The model under review builds one solid part; all positions refer to its coordinate system, in mm. A direction names the side the tool comes from. Round coordinates to 2 decimals unless told otherwise and drop trailing zeros. Write each loop counter-clockwise with the first axis right and the second up, starting at its lowest first coordinate (ties: lowest second). Pieces come first, ordered by that corner, then holes. Notation, with made-up numbers: M 13.25,61.25 L 36.25,61.25 A24 cw 36.25,100.25 Z; hole C 30.5,17.5 d9. An arc over 180 degrees is marked long. One line per item, written item: value. Start each with the question number.
1) Wall thickness on probe 1 along Z at (x, y) = (0, -85); probe 2 along Y at (x, z) = (16, 29); probe 3 along X at (y, z) = (-97, -0.5): over which ranges is each line inside the solid? List them lowest first.
2) Mouldability with a two-part tool opening along Z and no side actions: class faces 3 (the face through (0, -30, 0)), 4 (the face through (-2.927, -69.44, -13.183)), 5 (the face through (51.884, -15.21, -53.401)), 6 (the face through (0, 0, -2)) as +Z half, -Z half, draft (parallel to the pull), parting line (faces both ways), or undercut.
3) For P1, Ø3, axis at x = 11, y = -62, coming from the -Z side; P2, Ø1.5, axis at y = -51.5, z = 2.5, coming from the -X side; P3, Ø4, axis at x = 6, y = -80, coming from the -Z side, all flat-tipped, find the tip position at first contact; note any pin that passes through.
4) Tool access review of faces 1 (the face through (51.962, -15.21, 48.431)), 2 (the face through (-6.68, -39.86, -30.08)): name each direction out of +Z, -Z, +X, -X, +Y, -Y from which nothing blocks a thin tool from reaching the whole face with its end or side.
5) Take a section at D-D, the plane z = -22. Write out the cut boundary in (x, y), and give its area (3 significant figures).
6) Take a section at B-B, the plane x = 0. Write out the cut boundary in (y, z), and give its area (3 significant figures).
7) Take a section at A-A, the plane z = 0. Write out the cut boundary in (x, y), and give its area (3 significant figures).
8) Take a section at C-C, the plane y = -99.5. Write out the cut boundary in (x, z).
from build123d import *

# Parameters (mm, degrees)
F0_W     = 105.912518
F0_H     = 104.761295
F1_DEPTH = 30
F2_R     = 5
F3_R     = 30.813713
F3_R_2   = 23.380782
F4_DEPTH = 20
F5_R     = 23.490351
F5_R_2   = 13.503853
F6_DEPTH = 80


with BuildPart() as f1:
    # F0 (on Front) → F1 (new body)
    with BuildSketch(Plane.XZ):
        with Locations((0.431707, -2.446345)):
            Rectangle(F0_W, F0_H)
    extrude(amount=F1_DEPTH)

    # F2
    f2_edges = [f1.edges().sort_by_distance(p)[0] for p in [
        (53.387966, -15, 49.934302),
        (53.387966, -15, -54.826993),
        (-52.524552, -15, 49.934302),
        (-52.524552, -15, -54.826993),
    ]]
    fillet(f2_edges, radius=F2_R)

    # F3 (on face) → F4 (join)
    with BuildSketch(Plane.XZ.offset(30)):
        Circle(F3_R)
        Circle(F3_R_2, mode=Mode.SUBTRACT)
    extrude(amount=F4_DEPTH)

    # F5 (on face) → F6 (join)
    with BuildSketch(Plane.XZ.offset(30)):
        Circle(F5_R)
        Circle(F5_R_2, mode=Mode.SUBTRACT)
    extrude(amount=F6_DEPTH)


solid = f1.part
Checked values:
1. probe 1: z = -23.49 to -13.5, 13.5 to 23.49
1. probe 2: y = -30 to 0
1. probe 3: x = -23.49 to -13.49, 13.49 to 23.49
2. face 3: undercut
2. face 4: undercut
2. face 5: -Z half
2. face 6: draft
3. P1: stops at z = -21.48
3. P2: stops at x = -23.43
3. P3: stops at z = -23.15
4. face 1: +Z, +X, +Y, -Y
4. face 2: -Y
5. outline: M -52.52,-30 L -21.58,-30 L -21.58,-50 L -8.23,-50 L -8.23,-110 L 8.23,-110 L 8.23,-50 L 21.58,-50 L 21.58,-30 L 53.39,-30 L 53.39,0 L -52.52,0 Z
5. area: 5,030 mm2
6. outline: M -110,-23.49 L -50,-23.49 L -50,-30.81 L -30,-30.81 L -30,-54.83 L 0,-54.83 L 0,49.93 L -30,49.93 L -30,30.81 L -50,30.81 L -50,23.49 L -110,23.49 L -110,13.5 L -30,13.5 L -30,-13.5 L -110,-13.5 Z
6. area: 5,030 mm2
7. outline: M -52.52,-30 L -30.81,-30 L -30.81,-50 L -23.49,-50 L -23.49,-110 L -13.5,-110 L -13.5,-30 L 13.5,-30 L 13.5,-110 L 23.49,-110 L 23.49,-50 L 30.81,-50 L 30.81,-30 L 53.39,-30 L 53.39,0 L -52.52,0 Z
7. area: 5,070 mm2
8. outline: C 0,0 d46.98; hole C 0,0 d27.01
